Design review of the part built by this model. Coordinates are the model's own, in mm. Face numbers are marked on the shaded views. Give positions to 0.01 mm unless a question says otherwise; leave off trailing zeros. Loops run counter-clockwise (first coordinate to the right, second up) from the corner with the lowest first, then second, coordinate; pieces in that order, holes last. Notation, with made-up numbers: (17.5, -30) -> (66.5, -30) arc R35 ccw to (66.5, 5) -> close; hole circle Ø6 at (71, -8). An arc over 180 degrees is marked (long way). Use a Markdown table: item, result. Add a question column.
1. To check wall thickness, follow line 1 (Y direction, x = 0, z = -1); line 2 (Y direction, x = 0, z = 2); line 3 (X direction, y = 15.5, z = 0.25). State the ranges of each line that lie inside material, in increasing order.
2. Draft analysis for pull direction Y (two halves, no side actions). For the marked faces 1 and 2, state which applies: pulls with the +Y half, pulls with the -Y half, needs draft (parallel to the pull), parting line crosses it, or undercut.
3. Add section A-A (x = 0). State the section outline as (y, z) points (3 decimals).
4. For pin 1 Ø3 at (x, z) = (17.5, -2) entering from +Y, flat-tipped, find the tip position at first contact; note if it passes through.
```python
from build123d import *

# Parameters (mm, degrees)
F0_R        = 67
F0_R_2      = 59.6
F1_DEPTH    = 3.75
F2_R        = 63.875
F2_R_2      = 63.125
F3_DEPTH    = 1.5
F3_FACE_R   = 67
F3_FACE_R_2 = 63.875
F4_DEPTH    = 2
F4_TAPER    = -3
F7_DEPTH    = 6.5
F7_TAPER    = -3


# Not quite as in the source:
# - a feature of the source that left no trace in its solid (it failed there, or was rolled back) is left out


with BuildPart() as f1:
    # F0 (on Top) → F1 (new body, symmetric)
    with BuildSketch(Plane.XY):
        Circle(F0_R)
        Circle(F0_R_2, mode=Mode.SUBTRACT)
    extrude(amount=F1_DEPTH, both=True)

    # F2 (on face) → F3 (cut)
    with BuildSketch(Plane.XY.offset(3.75)):
        Circle(F2_R)
        Circle(F2_R_2, mode=Mode.SUBTRACT)
    extrude(amount=-F3_DEPTH, mode=Mode.SUBTRACT)

    # F3_face (on face) → F4 (cut)
    with BuildSketch(Plane.XY.offset(3.75)):
        Circle(F3_FACE_R)
        Circle(F3_FACE_R_2, mode=Mode.SUBTRACT)
    extrude(amount=-F4_DEPTH, taper=F4_TAPER, mode=Mode.SUBTRACT)

    # F6 (on face) → F7 (cut)
    with BuildSketch(Plane.XY.offset(3.75)):
        Polygon((61, 0.15), (59.4, 0.675), (59.4, -0.675), (61, -0.15), align=None)
    extrude(amount=-F7_DEPTH, taper=F7_TAPER, mode=Mode.SUBTRACT)


solid = f1.part
```
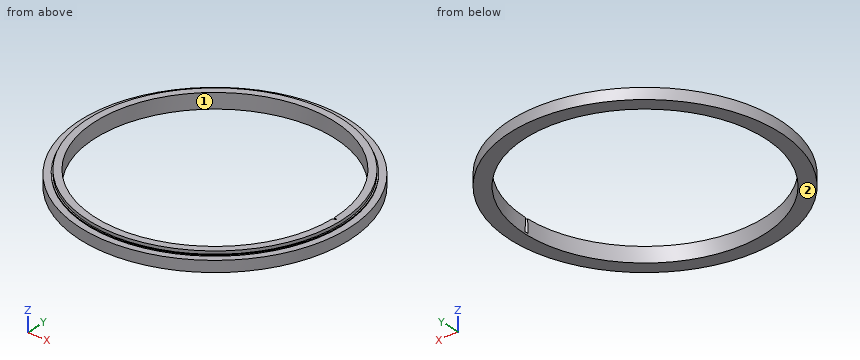
Taken from the geometry:
| question | item | result |
|---|---|---|
| 1 | line 1 | y = -67 to -59.6, 59.6 to 67 |
| 1 | line 2 | y = -63.78 to -59.6, 59.6 to 63.78 |
| 1 | line 3 | x = -65.18 to -57.55, 57.55 to 65.18 |
| 2 | face 1 | undercut |
| 2 | face 2 | needs draft |
| 3 | outline | (-67, -3.75) -> (-59.6, -3.75) -> (-59.6, 3.75) -> (-63.125, 3.75) -> (-63.125, 2.25) -> (-63.796, 2.25) -> (-63.77, 1.75) -> (-67, 1.75) -> close; (59.6, -3.75) -> (67, -3.75) -> (67, 1.75) -> (63.77, 1.75) -> (63.796, 2.25) -> (63.125, 2.25) -> (63.125, 3.75) -> (59.6, 3.75) -> close |
| 4 | pin 1 | stops at y = 65.06 |
